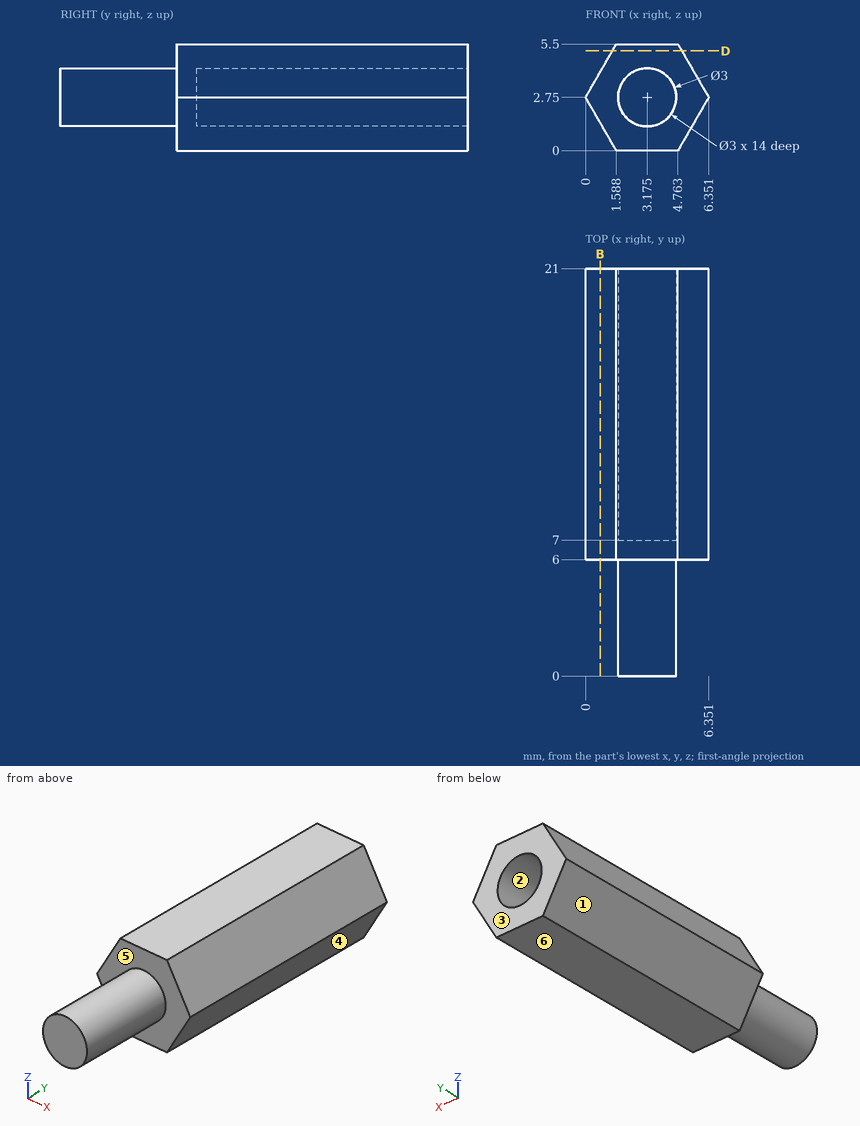
Verification items for this drawing (mm, ordinates from the low corner). A direction names the side the tool comes from. Round coordinates to 2 decimals unless told otherwise and drop trailing zeros. Order: outer loops, then holes, each group sorted by start corner. A loop starts at its lowest first (then second) coordinate and runs counter-clockwise, first axis right, second up. Notation, with made-up numbers: (-7.5, 36) - (40.5, 36) arc R30 cw to (40.5, 62) - close; hole circle Ø9 at (-1, 75.5). An arc over 180 degrees is marked (long way). Use CSV: the item, a comma, the result in double quotes.
(1) Access from +Z, -Z, +X, -X, +Y, -Y to the whole of each face (thin tool, end or side, straight path). Record for the marked faces 5 and 6.
Entries:
face 5,"-Y"
face 6,"-Z, +X, -X, +Y, -Y"
(2) Thickness scan on probe 1 along X at (y, z) = (18.75, 2.55) (1 decimal); probe 2 along X at (y, z) = (8.5, 1.9); probe 3 along Z at (x, y) = (2.5, 15.25). Record the ranges inside material, lowest first. Write a range as from..to.
Entries:
probe 1,"0.1..1.7, 4.7..6.2"
probe 2,"0.49..1.94, 4.41..5.86"
probe 3,"0..1.41, 4.09..5.5"
(3) Section check D-D on z = 5.15. Record the boundary of the cut face in (x, y) (1 decimal), and give its area (3 significant figures).
Entries:
outline,"(1.4, 6) - (5, 6) - (5, 21) - (1.4, 21) - close"
area,"53.7 mm^2"
(4) Mould release check, pull along X, two halves, no side actions. Record for the marked faces 1, 2, 3 and 4: released by +X, released by -X, zero draft, split by the parting line, or undercut.
Entries:
face 1,"released by -X"
face 2,"undercut"
face 3,"zero draft"
face 4,"released by +X"
(5) Gauge pin test, flat ends, axial feed: pin 1 Ø0.9 at (x, z) = (3, 2) entering from +Y; pin 2 Ø1.5 at (x, y) = (2.5, 4.5) entering from -Z; pin 3 Ø2 at (x, z) = (5.5, 1) entering from -Y. Record the tip position at first contact, or that the pin passes through.
Entries:
pin 1,"y = 7"
pin 2,"z = 1.25"
pin 3,"y = 6"
(6) Section check B-B on x = 0.75. Record the boundary of the cut face in (y, z).
Entries:
outline,"(6, 1.45) - (21, 1.45) - (21, 4.05) - (6, 4.05) - close"
